from build123d import *

# Parameters (mm, degrees)
F0_R     = 12.7
F1_DEPTH = 19.05


with BuildPart() as f1:
    # F0 (on Top) → F1 (new body)
    with BuildSketch(Plane.XY):
        with BuildLine():
            ThreePointArc((-166.801477, -133.35), (-166.801477, -146.05), (-155.802955, -152.4))
            Line((-155.802955, -152.4), (155.802955, -152.4))
            ThreePointArc((155.802955, -152.4), (166.801477, -146.05), (166.801477, -133.35))
            Line((166.801477, -133.35), (10.998523, 136.508634))
            ThreePointArc((10.998523, 136.508634), (0, 142.858634), (-10.998523, 136.508634))
            Line((-10.998523, 136.508634), (-166.801477, -133.35))
        make_face()
        with Locations((0, 95.25)):
            Circle(F0_R, mode=Mode.SUBTRACT)
    extrude(amount=F1_DEPTH)


solid = f1.part
Build history of the part. All positions in model axes, mm. Round coordinates to 2 decimals unless told otherwise and drop trailing zeros. Write each loop counter-clockwise with the first axis right and the second up, starting at its lowest first coordinate (ties: lowest second). Pieces come first, ordered by that corner, then holes. Notation, with made-up numbers: M 71.5,76.25 L 127.5,76.25 A18 ccw 127.5,89.25 Z; hole C -14.5,50 d3. An arc over 180 degrees is marked long. Answer as a JSON object with one key per item and string values. Group by question number.
(1) Drill centre lines: L1, parallel to Y at x = 0, z = 6.5; L2, parallel to Y at x = 6, z = 13.25; L3, parallel to X at y = -138.5, z = 6. Where is each one in solid material? Low to high.
(2) Cut at A-A (z = 11.75). Give the cut face in (x, y), and give its area (3 significant figures).
(3) Cut at B-B (x = 0). Give the cut face in (y, z), and give its area (3 significant figures).
(4) Flat gauge pins, fed straight in: pin 1 (1.5 mm diameter, centred on x = -20.5, z = 17, fed in from +Y); pin 2 (1.5 mm diameter, centred on y = -85.5, z = 8, fed in from -X); pin 3 (1.5 mm diameter, centred on y = 12, z = 12, fed in from -X). Where does each tip first touch, or does it go through?
(5) Cut at C-C (y = 95.25). Give the cut face in (x, z), and give its area (3 significant figures).
(6) Cut at D-D (x = 141.5). Give the cut face in (y, z), and give its area (3 significant figures).
(7) Mould opens along X. For faces 1 (the flat face through (-2, -68, 19.05)), 2 (the cylindrical face through (-2.75, 82.85, 9.39)), 3 (the cylindrical face through (166.707, -146.211, 9.392)) say: pulls with the +X half, pulls with the -X half, needs draft (parallel to the pull), parting line crosses it, or undercut.
Responses:
{
 "1": {"L1": "y = -152.4 to 82.55, 107.95 to 142.86", "L2": "y = -152.4 to 84.06, 106.44 to 141.35", "L3": "x = -168.45 to 168.45"},
 "2": {"outline": "M -166.8,-133.35 A12.7 ccw -155.8,-152.4 L 155.8,-152.4 A12.7 ccw 166.8,-133.35 L 11,136.51 A12.7 ccw -11,136.51 Z; hole C 0,95.25 d25.4", "area": "53,900 mm2"},
 "3": {"outline": "M -152.4,0 L 82.55,0 L 82.55,19.05 L -152.4,19.05 Z; M 107.95,0 L 142.86,0 L 142.86,19.05 L 107.95,19.05 Z", "area": "5,140 mm2"},
 "4": {"pin 1": "stops at y = 121.35", "pin 2": "stops at x = -139.61", "pin 3": "stops at x = -83.32"},
 "5": {"outline": "M -34.82,0 L -12.7,0 L -12.7,19.05 L -34.82,19.05 Z; M 12.7,0 L 34.82,0 L 34.82,19.05 L 12.7,19.05 Z", "area": "843 mm2"},
 "6": {"outline": "M -152.4,0 L -89.53,0 L -89.53,19.05 L -152.4,19.05 Z", "area": "1,200 mm2"},
 "7": {"face 1": "needs draft", "face 2": "undercut", "face 3": "pulls with the +X half"}
}
